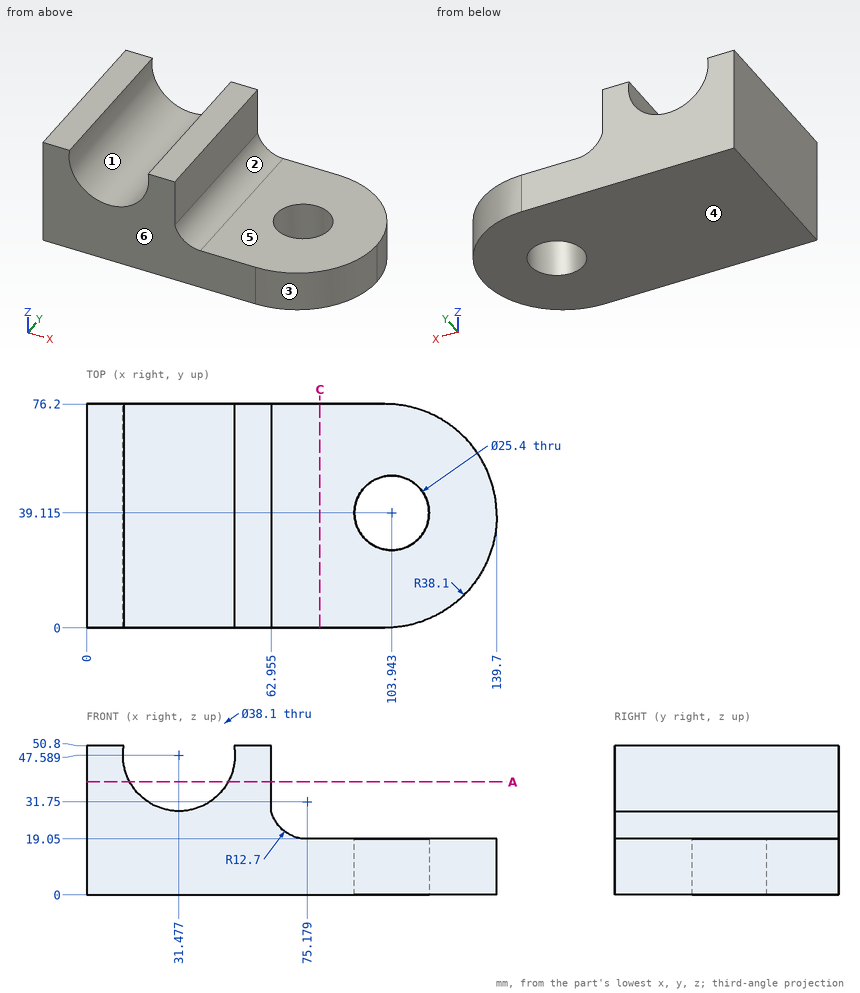
Job drawing, mm, ordinate dimensions from the low corner. One solid piece. A direction names the side the tool comes from. Give positions to 0.01 mm unless a question says otherwise; leave off trailing zeros. Loops run counter-clockwise (first coordinate to the right, second up) from the corner with the lowest first, then second, coordinate; pieces in that order, holes last. Notation, with made-up numbers: (28.5, 13) - (77.5, 13) arc R32 cw to (77.5, 40) - close; hole circle Ø9 at (74.5, 26.5). An arc over 180 degrees is marked (long way). Use one line per item in the form item = value.
(1) Pull direction Z, two halves, no side cores. Call the marked faces 1, 2, 3 and 4: pulls with the +Z half, pulls with the -Z half, needs draft (parallel to the pull), parting line crosses it, or undercut.
Determined:
face_1 = undercut
face_2 = pulls with the +Z half
face_3 = needs draft
face_4 = pulls with the -Z half
(2) Drill centre lines: L1, parallel to X at y = 38.5, z = 18; L2, parallel to X at y = 47, z = 14 (1 decimal); L3, parallel to Z at x = 133.5, y = 23. Where is each one in solid material? Low to high.
Determined:
L1 = 0 to 91.26, 116.63 to 139.7
L2 = 0 to 94, 113.9 to 138.6
L3 = 0 to 19.05
(3) Drop flat-ended pins along their axis: P1, Ø19.5, axis at x = 123, y = 52, coming from the +Z side; P2, Ø3, axis at y = 39.5, z = 25.5, coming from the +X side; P3, Ø18, axis at y = 48, z = 44.5, coming from the +X side (1 decimal); P4, Ø23, axis at x = 103.94, y = 39.12, coming from the +Z side. Give the stop position or say it passes through.
Determined:
P1 = 19.05
P2 = 65.12
P3 = 63
P4 = through
(4) Cut at C-C (x = 79.5). Give the cut face in (y, z), then the cut area to 3 significant figures.
Determined:
outline = (0, 0) - (76.2, 0) - (76.2, 19.05) - (0, 19.05) - close
area = 1,450 mm^2
(5) Cut at A-A (z = 38.5). Give the cut face in (x, y) (1 decimal).
Determined:
outline = (0, 0) - (14.7, 0) - (14.7, 76.2) - (0, 76.2) - close; (48.2, 0) - (63, 0) - (63, 76.2) - (48.2, 76.2) - close
(6) 3-axis set-ups, long thin cutter, end or side, ignore diameter. For the marked faces 5 and 6: which of +Z, -Z, +X, -X, +Y, -Y reach the whole face in a straight line?
Determined:
face_5 = +Z, +X, +Y, -Y
face_6 = +Z, -Z, +X, -X, -Y
